Here's how the part is built. I have some questions about the finished solid (model axes, mm). Face numbers are marked on the shaded views. A direction names the side the tool comes from. Give positions to 0.01 mm unless a question says otherwise; leave off trailing zeros. Write each loop counter-clockwise with the first axis right and the second up, starting at its lowest first coordinate (ties: lowest second). Pieces come first, ordered by that corner, then holes. Notation, with made-up numbers: (-30, -14.5) - (7, -14.5) arc R22 ccw to (7, 16.5) - close; hole circle Ø5 at (-27.5, -2). An arc over 180 degrees is marked (long way). Use a Markdown table: item, result.
Autodesk Inventor part; units mm, degrees
ref_plane "YZ Plane" through (0, 0, 0) normal (1, 0, 0) x (0, 1, 0)
ref_plane "XZ Plane" through (0, 0, 0) normal (0, 1, 0) x (-1, 0, 0)
ref_plane "XY Plane" through (0, 0, 0) normal (0, 0, 1) x (1, 0, 0)
sketch "Sketch1" plane through (0, 0, 0) normal (0, 0, 1) x (1, 0, 0)
  line L0 (-13.5571, -30) -> (11.7429, -30) construction
  line L1 (11.7429, -30) -> (11.7429, -13.7014) construction
  line L2 (11.7429, -13.7014) -> (-13.5571, -13.7014) construction
  line L3 (-13.5571, -13.7014) -> (-13.5571, -30) construction
  circle A0 centre (0, 0) radius 10
  circle A1 centre (0, 0) radius 23.5 construction
  line L4 (11.7429, -30) -> (21.2173, -10.1032) construction
  line L5 (-13.5571, -30) -> (-21.9053, -8.5093) construction
  circle A2 centre (0, 0) radius 27.5
  line L6 (-13.4496, -35) -> (13.2752, -35)
  line L7 (-13.4496, -35) -> (-24.6844, -12.1216)
  line L8 (13.2752, -35) -> (24.6094, -12.273)
  circle A3 centre (23.8157, 13.75) radius 5
  line L9 (-0.006, -0.0035) -> (23.8157, 13.75) construction
  line L10 (-0.006, -0.0035) -> (30.724, -0.0035) construction
  line L11 (-0.006, -0.0035) -> (23.8127, -13.7552) construction
  circle A4 centre (23.8127, -13.7552) radius 5
  circle A5 centre (23.8157, 13.75) radius 3.075
  circle A6 centre (23.8127, -13.7552) radius 3.075
  line L12 (-0.006, -0.0035) -> (-0.006, 21.9972)
  circle A7 centre (-23.8278, 13.75) radius 5
  circle A8 centre (-23.8248, -13.7552) radius 5
  circle A9 centre (-23.8278, 13.75) radius 3.075
  circle A10 centre (-23.8248, -13.7552) radius 3.075
  point P0 (20.9324, 17.8349)
  point P1 (-20.9369, 17.8296)
  point P2 (-25.9134, 9.2058)
  point P3 (-25.9114, -9.2114)
  point P4 (-21.6672, -18.2658)
  point P5 (21.6274, -18.2524)
  point P6 (25.9097, -9.2162)
  point P7 (25.9117, 9.2105)
  dimension "d0" = 25.3
  dimension "d1" = 20
  dimension "d2" = 30
  dimension "d3" = 47
  dimension "d4" = 55
  dimension "d5" = 5
  dimension "d45" = 30
  dimension "d46" = 10
  dimension "d47" = 30
  dimension "d48" = 10
  dimension "d49" = 6.15
  dimension "d50" = 6.15
  dimension "d64" = 6.15
extrude "Extrusion1" add sketch "Sketch1" along normal blind 4 contours A2 A4 A8 A7 A3 | A3 A2 A5 | A2 A5 A3 | A4 L8 A6 A2 | A2 A6 A4 | A4 L8 L6 L7 A8 A2 | A2 A6 L8 A4 | A7 A2 A9 | A2 A9 A7 | A8 L7 A10 A2 | A2 A10 A8 | A8 A2 A10 L7
sketch "Sketch2" plane through (0, 0, 4) normal (0, 0, 1) x (1, 0, 0)
  line L0 (-21.6672, -18.2658) -> (-13.4496, -35)
  line L1 (-13.4496, -35) -> (-15.4139, -31)
  line L2 (15.2701, -31) -> (-15.4139, -31)
  line L3 (13.2752, -35) -> (21.6274, -18.2524)
  line L4 (15.2701, -31) -> (13.2752, -35)
  line L5 (-13.4496, -35) -> (13.2752, -35)
  line L6 (-13.4496, -35) -> (13.2752, -35)
  point P0 (0, 0)
  point P1 (-24.6844, -12.1216)
  point P2 (24.6094, -12.273)
  dimension "d8" = 4
extrude "Extrusion2" add sketch "Sketch2" along normal blind 25
sketch "Sketch3" plane through (0, 0, 29) normal (0, 0, 1) x (1, 0, 0)
  line L0 (-13.5571, -30) -> (11.7429, -30) construction
  line L1 (11.7429, -30) -> (11.7429, -13.7014) construction
  line L2 (11.7429, -13.7014) -> (-13.5571, -13.7014) construction
  line L3 (-13.5571, -13.7014) -> (-13.5571, -30) construction
  circle A0 centre (0, 0) radius 10
  circle A1 centre (0, 0) radius 23.5 construction
  line L4 (11.7429, -30) -> (21.2173, -10.1032) construction
  line L5 (-13.5571, -30) -> (-21.9053, -8.5093) construction
  circle A2 centre (0, 0) radius 27.5
  line L6 (-13.4496, -35) -> (13.2752, -35)
  line L7 (-13.4496, -35) -> (-24.6844, -12.1216)
  line L8 (13.2752, -35) -> (24.6094, -12.273)
  circle A3 centre (23.8157, 13.75) radius 5
  line L9 (-0.006, -0.0035) -> (23.8157, 13.75) construction
  line L10 (-0.006, -0.0035) -> (30.724, -0.0035) construction
  line L11 (-0.006, -0.0035) -> (23.8127, -13.7552) construction
  circle A4 centre (23.8127, -13.7552) radius 5
  circle A5 centre (23.8157, 13.75) radius 3.125
  circle A6 centre (23.8127, -13.7552) radius 3.125
  line L12 (-0.006, -0.0035) -> (-0.006, 21.9972)
  circle A7 centre (-23.8278, 13.75) radius 5
  circle A8 centre (-23.8278, 13.75) radius 3.125
  circle A9 centre (-23.8248, -13.7552) radius 5
  circle A10 centre (-23.8248, -13.7552) radius 3.125
  circle A11 centre (0, 0) radius 10
  point P0 (-42.8581, 50.0798)
  point P1 (-84.7274, 50.0745)
  point P2 (-89.7039, 41.4507)
  point P3 (-89.7018, 23.0335)
  point P4 (-85.4577, 13.9792)
  point P5 (-42.163, 13.9925)
  point P6 (-37.8808, 23.0287)
  point P7 (-37.8788, 41.4554)
  point P8 (20.9324, 17.8349)
  point P9 (-20.9369, 17.8296)
  point P10 (-25.9134, 9.2058)
  point P11 (-25.9114, -9.2114)
  point P12 (-21.6672, -18.2658)
  point P13 (21.6274, -18.2524)
  point P14 (20.9285, -17.8395)
  point P15 (22.0984, -16.368)
  point P16 (25.2195, -10.9648)
  point P17 (25.9117, 9.2105)
  point P18 (25.9097, -9.2162)
  dimension "d51" = 25.3
  dimension "d52" = 20
  dimension "d53" = 30
  dimension "d54" = 47
  dimension "d55" = 55
  dimension "d56" = 5
  dimension "d57" = 30
  dimension "d58" = 10
  dimension "d59" = 30
  dimension "d60" = 10
  dimension "d61" = 6.25
  dimension "d62" = 6.25
extrude "Extrusion3" add sketch "Sketch3" along normal blind 4 contours A2 A4 A9 A7 A3 | A3 A2 A5 | A2 A5 A3 | A4 L8 A6 A2 | A2 A6 A4 | A4 L8 L6 L7 A9 A2 | A2 A6 L8 A4 | A7 A2 A8 | A2 A8 A7 | A9 L7 A10 A2 | A2 A10 A9 | A9 A2 A10 L7
sketch "Sketch4" plane through (0, 0, 0) normal (1, 0, 0) x (0, 1, 0)
  line L0 (-31, 4) -> (-31, 29)
  line L1 (16.3793, 67.7391) -> (20.3793, 67.7391) construction
  line L2 (20.3793, 44.4757) -> (20.3793, 67.7391) construction
  line L3 (20.3793, 44.4757) -> (16.3793, 44.4757) construction
  line L4 (0, 24) -> (0, 4)
  line L5 (16.3793, 44.4757) -> (16.3793, 48.4757) construction
  line L6 (16.3793, 67.7391) -> (16.3793, 63.7391) construction
  arc A0 (16.3793, 63.7391) -> (16.3793, 48.4757) centre (22.0199, 56.1074) ccw construction
  line L7 (27.5, 4) -> (17.8296, 4)
  line L8 (27.5, 29) -> (27.5, 33)
  line L9 (27.5, 29) -> (-12.273, 29)
  line L10 (27.5, 29) -> (25, 29)
  line L11 (25, 29) -> (25, 22.5)
  arc A1 (25, 22.5) -> (25, 10.5) centre (31.0208, 16.5) ccw
  line L12 (25, 10.5) -> (25, 4)
  line L13 (27.5, 4) -> (25, 4)
  line L14 (25, 29) -> (27.5, 29)
  line L15 (27.5, 4) -> (27.5, 29)
  line L16 (27.5, 4) -> (17.8296, 4)
  line L17 (27.5, 4) -> (25, 4)
  point P0 (0, 0)
  point P1 (-12.1216, 29)
  point P2 (-12.1216, 4)
  point P3 (-12.273, 29)
  point P4 (25, 7.25)
  point P5 (17.8349, 4)
  point P6 (9.2058, 4)
  point P7 (-9.2114, 4)
  dimension "d22" = 4
  dimension "d23" = 4
  dimension "d24" = 4
  dimension "d26" = 6.5
  dimension "d28" = 6.5
  dimension "d65" = 2.5
  dimension "d66" = 2.5
revolve "Revolution1" add sketch "Sketch4" angle 80 mid plane about axis through (0, 0, 24) along (0, 0, -1)
sketch "Sketch5" plane through (0, 0, 0) normal (0, 1, 0) x (-1, 0, 0)
  line L0 (0, 0) -> (0.0872, 33)
sketch "Sketch7" plane through (0, 0, 0) normal (1, 0, 0) x (0, 1, 0)
  line L0 (29.2747, 11.9493) -> (29.2747, 21.0264) construction
  ellipse E0 centre (23.7633, 16.5) end of major axis (23.7633, 8) minor radius 6.5114 (19.1511, 22.5) -> (19.1511, 10.5) ccw
  line L1 (29.2747, 16.4878) -> (30.2747, 16.4878)
  arc A0 (29.2747, 11.9493) -> (29.2747, 21.0264) centre (45.8325, 16.4878) ccw
  arc A1 (30.2415, 15.6424) -> (30.2747, 16.4878) centre (23.4449, 16.3328) ccw
  line L2 (29.2747, 21.0264) -> (27.6139, 21.0264)
  line L3 (27.6139, 21.0264) -> (27.6139, 13.9093)
  line L4 (27.6139, 13.9093) -> (29.2747, 13.9093)
  line L5 (29.2747, 13.9093) -> (29.2747, 21.0264)
  point P0 (0, 0)
  point P1 (13.8599, 14.7128)
  point P2 (13.8237, 14.0101)
  point P3 (14.8237, 10.4516)
  dimension "d29" = 1
extrude "Extrusion4" [suppressed]
sketch "Sketch9" plane through (-13.4496, -35, 0) normal (0, -1, 0) x (1, 0, 0)
  circle A0 centre (13.3624, 16.5) radius 5
  line L0 (0, 33) -> (26.7249, 33)
  line L1 (0, 0) -> (0, 29)
  line L2 (26.7249, 0) -> (26.7249, 29)
  line L3 (0, 0) -> (26.7249, 0)
  point P0 (13.4496, 0)
  dimension "d34" = 16.5
  dimension "d35" = 13.3624
  dimension "d36" = 26.7249
  dimension "d37" = 10
  dimension "d44" = 33
extrude "Extrusion5" cut sketch "Sketch9" against normal up to surface (4 mm away)
ref_plane "Work Plane1" through (16.0697, 19.1511, 29) normal (-1, 0, 0) x (0, 0, -1)
sketch "Sketch11" plane through (0, 0, 33) normal (0, 0, 1) x (1, 0, 0)
  point P0 (0, 0)
fillet "Fillet3" radius 6 14 edges at (20.9324, 17.8349, 31) (20.9324, 17.8349, 2) (25.9117, 9.2105, 31) (25.9117, 9.2105, 2) (25.9097, -9.2162, 2) (21.6274, -18.2524, 2) (-25.9134, 9.2058, 31) (-25.9134, 9.2058, 2) (-20.9369, 17.8296, 2) (-20.9369, 17.8296, 31) (-25.9114, -9.2114, 31) (-21.6672, -18.2658, 31) (25.9097, -9.2162, 31) (21.6274, -18.2524, 31)
equation "\"d35\" = 0.5 * d36"
properties part number "pulleyblocker"
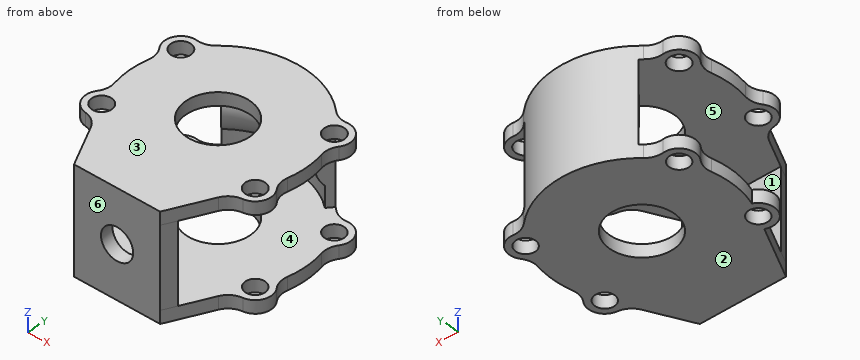
Item 1: If we section it at A-A, the plane y = 0: Write out the boundary of the cut face in (x, z), plus the area to 3 significant figures.
Values:
| item | result |
|---|---|
| outline | (-27.5, 0) - (-10, 0) - (-10, 4) - (-27.5, 4) - close; (-27.5, 29) - (-10, 29) - (-10, 33) - (-27.5, 33) - close; (10, 0) - (27.5, 0) - (27.5, 4) - (10, 4) - close; (10, 29) - (27.5, 29) - (27.5, 33) - (10, 33) - close |
| area | 280 mm2 |
Item 2: For the marked faces 1 and 2, which set-ups out of +Z, -Z, +X, -X, +Y, -Y let a thin tool reach every point of the face, with its end or its side?
Values:
| item | result |
|---|---|
| face 1 | +X, -X |
| face 2 | -Z, +X, -X, +Y, -Y |
Item 3: If we section it at D-D, the plane y = -25.5: Write out the boundary of the cut face in (x, z), plus the area to 3 significant figures.
Values:
| item | result |
|---|---|
| outline | (-18.11, 0) - (18.01, 0) - (18.01, 4) - (-18.11, 4) - close; (-18.11, 29) - (18.01, 29) - (18.01, 33) - (-18.11, 33) - close |
| area | 289 mm2 |
Item 4: If we section it at B-B, the plane y = 13.75: Write out the boundary of the cut face in (x, z), plus the area to 3 significant figures.
Values:
| item | result |
|---|---|
| outline | (-28.83, 0) - (-26.9, 0) - (-26.9, 4) - (-28.83, 4) - close; (-28.83, 29) - (-26.95, 29) - (-26.95, 33) - (-28.83, 33) - close; (-20.75, 0) - (20.74, 0) - (20.74, 4) - (-20.75, 4) - close; (-20.7, 29) - (20.69, 29) - (20.69, 33) - (-20.7, 33) - close; (26.89, 0) - (28.82, 0) - (28.82, 4) - (26.89, 4) - close; (26.94, 29) - (28.82, 29) - (28.82, 33) - (26.94, 33) - close |
| area | 362 mm2 |
Item 5: Will these pins go through, and if not, where does the flat tip stop? pin 1 Ø10 at (x, z) = (-21, 5) entering from +Y; pin 2 Ø5.5 at (x, y) = (23.82, 13.75) entering from -Z; pin 3 Ø3 at (x, z) = (-4.5, 14.5) entering from +Y; pin 4 Ø6 at (y, z) = (-0.5, 4) entering from +X.
Values:
| item | result |
|---|---|
| pin 1 | stops at y = 22.37 |
| pin 2 | passes through |
| pin 3 | stops at y = 27.34 |
| pin 4 | stops at x = 27.5 |
Item 6: If we section it at C-C, the plane z = 16.5: Write out the boundary of the cut face in (x, y), plus the area to 3 significant figures.
Values:
| item | result |
|---|---|
| outline | (-17.68, 21.07) - (-14.48, 17.25) arc R22.52 cw to (14.48, 17.25) - (17.68, 21.07) arc R27.5 ccw to start; (-15.41, -31) - (-13.45, -35) - (-5.09, -35) - (-5.09, -31) - close; (4.91, -35) - (13.28, -35) - (15.27, -31) - (4.91, -31) - close |
| area | 249 mm2 |
Item 7: I need wall thicknesses on line 1 along X through (y, z) = (13.75, 0.8); line 2 along Z through (x, y) = (-5.5, -23.5); line 3 along X through (y, z) = (13.75, 30.95). Which ranges of each line are inside material? Lowest first, please. Write a range as [from, to].
Values:
| item | result |
|---|---|
| line 1 | x = [-28.83, -26.9], [-20.75, 20.74], [26.89, 28.82] |
| line 2 | z = [0, 4], [29, 33] |
| line 3 | x = [-28.83, -26.95], [-20.7, 20.69], [26.94, 28.82] |
Item 8: Thinking about a two-plate mould opening in Z: for the marked faces 3, 4, 5 and 6, which applies, +Z half, -Z half, draft (parallel to the pull), parting line (faces both ways), or undercut?
Values:
| item | result |
|---|---|
| face 3 | +Z half |
| face 4 | undercut |
| face 5 | undercut |
| face 6 | draft |
